Check sheet for the modelled part. Datum: model origin and axes. Units: mm. A direction names the side the tool comes from. Round coordinates to 2 decimals unless told otherwise and drop trailing zeros. Order: outer loops, then holes, each group sorted by start corner. A loop starts at its lowest first (then second) coordinate and runs counter-clockwise, first axis right, second up.
Q1. Depth check by flat-ended pin: P1, Ø8, axis at x = 34.5, y = 31.5, coming from the +Z side; P2, Ø1.5, axis at x = 6, y = -23, coming from the +Z side; P3, Ø4, axis at x = -15.5, y = -54, coming from the -Z side. Enter the tip coordinate at first touch or a pass-through.
Q2. Mould release check, pull along Y, two halves, no side actions. Record for faces 1 (the conical face through (-16.3, -62.38, 31.33)), 2 (the cylindrical face through (14.28, 33.96, 64.32)), 3 (the flat face through (30, -46.454, 9)): +Y half, -Y half, draft (parallel to the pull), parting line (faces both ways), or undercut.
Q3. Cross-section at B-B on z = 0. Record the cut outline in (x, y).
Q4. Cross-section at A-A on x = 0. Record the cut outline in (y, z), then the cut area to 3 significant figures.
Q5. Scan lines: probe 1 along X at (y, z) = (-4, 0); probe 2 along X at (y, z) = (-83, -15.5). Record each from-to range of solid material in increasing order.
Q6. Cross-section at D-D on y = 29. Record the cut outline in (x, z), then the cut area to 3 significant figures.
Q7. Set-up check for faces 4 (the flat face through (0, 34.138, -40)), 5 (the flat face through (22, 8.738, -48)), 6 (the flat face through (-21, 21.438, 63)), 7 (the cylindrical face through (71.37, 15, -3.14)), 8 (the flat face through (0.2, -102.391, 46.3)): record each of +Z, -Z, +X, -X, +Y, -Y from which the full face is reachable in a straight line by a thin tool's end or side.
Autodesk Inventor part; units mm, degrees
ref_plane "YZ Plane" through (0, 0, 0) normal (1, 0, 0) x (0, 1, 0)
ref_plane "XZ Plane" through (0, 0, 0) normal (0, 1, 0) x (-1, 0, 0)
ref_plane "XY Plane" through (0, 0, 0) normal (0, 0, 1) x (1, 0, 0)
sketch "Sketch1" plane through (0, 0, 0) normal (0, 0, 1) x (1, 0, 0)
  arc A0 (-19.4827, -3.287) -> (-19.05, 0) centre (-31.75, 0) ccw
  line L0 (-19.4827, -3.287) -> (-58.7375, -149.7878)
  line L1 (-65.8876, 46.8376) -> (-65.8876, 21.4376)
  line L2 (-65.8876, 21.4376) -> (-71.4375, 21.4376)
  line L3 (-44.45, 34.1376) -> (-38.6524, 34.1376)
  line L4 (-44.45, 34.1376) -> (0, 34.1376) construction
  line L5 (-37.3992, -46.4536) -> (-31.0492, -46.4536)
  line L6 (-71.4375, 21.4376) -> (-71.4375, 8.7376)
  line L7 (-71.4375, 8.7376) -> (-58.7375, 8.7376)
  line L8 (-58.7375, 8.7376) -> (-52.3875, 8.7376)
  line L9 (-52.3875, 8.7376) -> (-52.3875, -102.3907)
  line L10 (-71.4375, 8.7376) -> (-71.4375, -0.7874)
  line L11 (-71.4375, 8.7376) -> (-61.9125, 8.7376) construction
  line L12 (-71.4375, -0.7874) -> (-58.7375, -0.7874)
  line L13 (-58.7375, -0.7874) -> (-58.7375, -51.5874)
  line L14 (-58.7375, -51.5874) -> (-71.4375, -51.5874)
  line L15 (-71.4375, -0.7874) -> (-65.0875, -0.7874)
  line L16 (-65.0875, -0.7874) -> (-65.0875, -6.731)
  line L17 (-65.0875, -6.731) -> (-71.4375, -6.731)
  line L18 (-71.4375, 21.4376) -> (-71.4375, -0.7874)
  line L19 (-71.4375, -6.731) -> (-71.4375, -51.5874)
  line L20 (-58.7375, -51.5874) -> (-58.7375, -126.0892)
  line L21 (-58.7375, -51.5874) -> (0, -51.5874) construction
  line L22 (-46.0375, -102.3907) -> (-52.3875, -102.3907)
  line L23 (-65.0875, -51.5907) -> (-58.7375, -51.5907)
  line L24 (-58.7375, -149.7878) -> (-61.9125, -161.637)
  line L25 (-58.7375, -149.7878) -> (-34.203, -149.7878) construction
  line L26 (-65.0875, -161.637) -> (-61.9125, -161.637)
  line L27 (-58.7375, -126.0892) -> (-52.3875, -126.0892)
  line L28 (0, 34.1376) -> (0, 0)
  line L29 (-65.0875, -100.6892) -> (-65.0875, -161.637)
  line L30 (-58.7375, -51.5907) -> (-61.9125, -51.5907)
  line L31 (-65.0875, -100.6892) -> (-58.7375, -100.6892)
  line L32 (-65.8876, 46.8376) -> (-18.3062, 46.8376) construction
  line L33 (-65.8876, 46.8376) -> (-14.7047, 46.8376) construction
  line L34 (-65.8876, 46.8376) -> (-33.5957, 31.7796)
  line L35 (-65.8876, 46.8376) -> (-30.2574, 46.8376) construction
  arc A1 (-19.05, 0) -> (-33.5957, 31.7796) centre (-61.0391, 0) ccw
  line L36 (-44.45, 34.1376) -> (-44.45, -46.4536)
  line L37 (-44.45, 34.1376) -> (36.1412, 34.1376) construction
  line L38 (-44.45, -46.4536) -> (-37.3992, -46.4536)
  dimension "d86" = 19.05
  dimension "d87" = 25.4
  dimension "d88" = 5.5499
  dimension "d89" = 65.8876
  dimension "d90" = 12.7
  dimension "d91" = 12.7
  dimension "d92" = 44.45
  dimension "d93" = 6.35
  dimension "d94" = 105
  dimension "d95" = 12.7
  dimension "d96" = 12.7
  dimension "d97" = 6.35
  dimension "d98" = 9.525
  dimension "d99" = 50.8
  dimension "d100" = 12.7
  dimension "d101" = 6.35
  dimension "d102" = 5.9436
  dimension "d103" = 6.35
  dimension "d104" = 50.8
  dimension "d105" = 6.35
  dimension "d106" = 105
  dimension "d107" = 3.175
  dimension "d108" = 6.35
  dimension "d109" = 60.9478
  dimension "d110" = 3.175
  dimension "d111" = 6.35
  dimension "d112" = 25.4
  dimension "d113" = 25
  dimension "d114" = 41.9891
  dimension "d115" = 32.2919
  dimension "d116" = 90
  dimension "d117" = 80.5912
revolve "Revolution1" add sketch "Sketch1" angle 360 about axis through (0, 34.1376, 0) along (0, -1, 0) contours L0 L22 L9 L8 L7 L6 L2 L1 L34 L3 L36 L38 L5
properties part number "Phenolic" material "Phenolic Resin"
Results found:
1. P1: stops at z = 58.4
1. P2: stops at z = 52.12
1. P3: stops at z = -50.62
2. face 1: -Y half
2. face 2: draft
2. face 3: undercut
3. outline: (-71.44, 8.74) - (-52.39, 8.74) - (-52.39, -102.39) - (-46.04, -102.39) - (-31.05, -46.45) - (-44.45, -46.45) - (-44.45, 34.14) - (-38.65, 34.14) - (-65.89, 46.84) - (-65.89, 21.44) - (-71.44, 21.44) - close; (31.05, -46.45) - (46.04, -102.39) - (52.39, -102.39) - (52.39, 8.74) - (71.44, 8.74) - (71.44, 21.44) - (65.89, 21.44) - (65.89, 46.84) - (38.65, 34.14) - (44.45, 34.14) - (44.45, -46.45) - close
4. outline: (-102.39, -52.39) - (8.74, -52.39) - (8.74, -71.44) - (21.44, -71.44) - (21.44, -65.89) - (46.84, -65.89) - (34.14, -38.65) - (34.14, -44.45) - (-46.45, -44.45) - (-46.45, -31.05) - (-102.39, -46.04) - close; (-102.39, 46.04) - (-46.45, 31.05) - (-46.45, 44.45) - (34.14, 44.45) - (34.14, 38.65) - (46.84, 65.89) - (21.44, 65.89) - (21.44, 71.44) - (8.74, 71.44) - (8.74, 52.39) - (-102.39, 52.39) - close
4. area: 4,000 mm2
5. probe 1: x = -52.39 to -44.45, 44.45 to 52.39
5. probe 2: x = -50.04 to -37.79, 37.79 to 50.04
6. outline: circle Ø131.78 at (0, 0); hole circle Ø88.9 at (0, 0)
6. area: 7,430 mm2
7. face 4: none
7. face 5: -Y
7. face 6: +Y
7. face 7: +Y, -Y
7. face 8: +Z, -Z, +X, -X, -Y
